Here's how the part is built. I have some questions about the finished solid (model axes, mm). A direction names the side the tool comes from. Round coordinates to 2 decimals unless told otherwise and drop trailing zeros. Order: outer loops, then holes, each group sorted by start corner. A loop starts at its lowest first (then second) coordinate and runs counter-clockwise, first axis right, second up.
```python
from build123d import *

# Parameters (mm, degrees)
ESQUISSE1_W             = 165
ESQUISSE1_H             = 276
BOSS_EXTRU_1_DEPTH      = 6
ESQUISSE2_W             = 38
ESQUISSE2_H             = 6
ESQUISSE2_W_2           = 6
ESQUISSE2_H_2           = 32
ESQUISSE2_H_3           = 68
ESQUISSE2_W_3           = 40
EXTERIEUR_DEPTH         = 10
ESQUISSE3_R             = 11
ESQUISSE3_W             = 20
ESQUISSE3_H             = 6
ENL_V_MAT_EXTRU_2_DEPTH = 322.616230934
ESQUISSE4_R             = 1.5
ESQUISSE4_R_2           = 1.252769876
ESQUISSE4_R_3           = 1.193016672
ESQUISSE4_R_4           = 1.226747293
ESQUISSE4_R_5           = 1.185631844
ENL_V_MAT_EXTRU_3_DEPTH = 322.616230934
ESQUISSE5_R             = 2.995
ESQUISSE5_R_2           = 3
ESQUISSE5_R_3           = 2
ENL_V_MAT_EXTRU_4_DEPTH = 3
ESQUISSE6_W             = 20
ESQUISSE6_H             = 100
ENL_V_MAT_EXTRU_5_DEPTH = 322.616230934


with BuildPart() as part:
    # Esquisse1 → Boss.-Extru.1 (new body)
    with BuildSketch(Plane.XY):
        with Locations((-82.5, 138)):
            Rectangle(ESQUISSE1_W, ESQUISSE1_H)
    extrude(amount=BOSS_EXTRU_1_DEPTH)

    # Esquisse2 → exterieur (cut)
    with BuildSketch(Plane.XY.offset(6)):
        with Locations((-86, 273)):
            Rectangle(ESQUISSE2_W, ESQUISSE2_H)
        with Locations((-162, 220)):
            Rectangle(ESQUISSE2_W_2, ESQUISSE2_H_2)
        with Locations((-162, 102)):
            Rectangle(ESQUISSE2_W_2, ESQUISSE2_H_3)
        Polygon((-137, 36), (-137, 6), (-100, 6), (-100, 0), (-165, 0), (-165, 36), align=None)
        with Locations((-40, 3)):
            Rectangle(ESQUISSE2_W_3, ESQUISSE2_H)
    extrude(amount=-EXTERIEUR_DEPTH, mode=Mode.SUBTRACT)

    # Esquisse3 → Enlèv. mat.-Extru.2 (cut, through all)
    with BuildSketch(Plane.XY.offset(6)):
        with Locations((-144, 178.92)):
            Circle(ESQUISSE3_R)
        with Locations((-135, 99)):
            Rectangle(ESQUISSE3_W, ESQUISSE3_H)
    extrude(amount=-ENL_V_MAT_EXTRU_2_DEPTH, mode=Mode.SUBTRACT)

    # Esquisse4 → Enlèv. mat.-Extru.3 (cut, through all)
    with BuildSketch(Plane.XY.offset(6)):
        with Locations((-60, 273)):
            Circle(ESQUISSE4_R)
        with Locations((-112, 273)):
            Circle(ESQUISSE4_R)
        with Locations((-162, 197)):
            Circle(ESQUISSE4_R)
        with Locations((-162, 170)):
            Circle(ESQUISSE4_R)
        with Locations((-162, 143)):
            Circle(ESQUISSE4_R)
        with Locations((-162, 61)):
            Circle(ESQUISSE4_R)
        with Locations((-162, 43)):
            Circle(ESQUISSE4_R)
        with Locations((-93, 3)):
            Circle(ESQUISSE4_R)
        with Locations((-67, 3)):
            Circle(ESQUISSE4_R)
        with Locations((-10, 3)):
            Circle(ESQUISSE4_R)
        with Locations((-162, 269)):
            Circle(ESQUISSE4_R)
        with Locations((-162, 243)):
            Circle(ESQUISSE4_R)
        with Locations((-117.5, 27)):
            Circle(ESQUISSE4_R_2)
        with Locations((-117.5, 43)):
            Circle(ESQUISSE4_R_3)
        with Locations((-101.5, 43)):
            Circle(ESQUISSE4_R_4)
        with Locations((-101.5, 27)):
            Circle(ESQUISSE4_R_5)
        with Locations((-152, 99)):
            Circle(ESQUISSE4_R)
    extrude(amount=-ENL_V_MAT_EXTRU_3_DEPTH, mode=Mode.SUBTRACT)

    # Esquisse5 → Enlèv. mat.-Extru.4 (cut)
    with BuildSketch(Plane(origin=(0, 0, 0), x_dir=(-1, 0, 0), z_dir=(0, 0, -1))):
        with Locations((60, 273)):
            Circle(ESQUISSE5_R)
        with Locations((112, 273)):
            Circle(ESQUISSE5_R)
        with Locations((162, 197)):
            Circle(ESQUISSE5_R)
        with Locations((162, 170)):
            Circle(ESQUISSE5_R)
        with Locations((162, 143)):
            Circle(ESQUISSE5_R)
        with Locations((162, 61)):
            Circle(ESQUISSE5_R)
        with Locations((162, 43)):
            Circle(ESQUISSE5_R)
        with Locations((93, 3)):
            Circle(ESQUISSE5_R)
        with Locations((67, 3)):
            Circle(ESQUISSE5_R)
        with Locations((10, 3)):
            Circle(ESQUISSE5_R)
        with Locations((162, 269)):
            Circle(ESQUISSE5_R)
        with Locations((162, 243)):
            Circle(ESQUISSE5_R)
        with Locations((152, 99)):
            Circle(ESQUISSE5_R_2)
        with Locations((117.5, 43)):
            Circle(ESQUISSE5_R_3)
        with Locations((117.5, 27)):
            Circle(ESQUISSE5_R_3)
        with Locations((101.5, 27)):
            Circle(ESQUISSE5_R_3)
        with Locations((101.5, 43)):
            Circle(ESQUISSE5_R_3)
    extrude(amount=-ENL_V_MAT_EXTRU_4_DEPTH, mode=Mode.SUBTRACT)

    # Esquisse6 → Enlèv. mat.-Extru.5 (cut, through all)
    with BuildSketch(Plane(origin=(0, 0, 0), x_dir=(-1, 0, 0), z_dir=(0, 0, -1))):
        with Locations((107, 121)):
            Rectangle(ESQUISSE6_W, ESQUISSE6_H)
    extrude(amount=-ENL_V_MAT_EXTRU_5_DEPTH, mode=Mode.SUBTRACT)


solid = part.part
```
1) For faces 1 (the flat face through (-163.3, 241.7, 3)), 2 (the flat face through (-135, 276, 3)), 3 (the flat face through (-86, 270, 3)), 4 (the flat face through (-151, 36, 3)), which set-ups out of +Z, -Z, +X, -X, +Y, -Y let a thin tool reach every point of the face, with its end or its side?
2) If we section it at B-B (z = 4.3): Give the number of separate pieces and of enclosed holes in the cut face, plus the area to 3 significant figures.
3) If we section it at A-A (y = 131): Write out the boundary of the cut face in (x, z), plus the area to 3 significant figures.
4) I'm going to push flat-ended pins straight in: pin 1 (3 mm diameter, centred on y = 94, z = 4, fed in from -X); pin 2 (3 mm diameter, centred on x = -161.5, y = 143.5, fed in from -Z); pin 3 (1 mm diameter, centred on x = -38.5, z = 4, fed in from -Y). Where does each tip first touch, or does it pass through?
5) We'd pull the mould along Y, two halves only. Please class faces 5 (the flat face through (-165, 256, 3)), 6 (the flat face through (-61.3, 271.7, 3)), 7 (the flat face through (-40, 6, 3)): +Y half, -Y half, draft (parallel to the pull), parting line (faces both ways), or undercut.
6) I need wall thicknesses on line 1 (X direction, y = 123.5, z = 4.3); line 2 (Y direction, x = -10, z = 4.7); line 3 (X direction, y = 215.5, z = 3.9). Which ranges of each line are inside material? Lowest first, please.
7) If we section it at C-C (x = -75): Write out the boundary of the cut face in (y, z), plus the area to 3 significant figures.
Solutions:
1. face 1: -Z
1. face 2: +Z, -Z, +X, -X, +Y
1. face 3: +Z, -Z, +Y
1. face 4: +Z, -Z, -X, -Y
2. separate pieces: 1
2. enclosed holes: 20
2. area: 40,600 mm2
3. outline: (-159, 0) - (-117, 0) - (-117, 6) - (-159, 6) - close; (-97, 0) - (0, 0) - (0, 6) - (-97, 6) - close
3. area: 834 mm2
4. pin 1: stops at x = -159
4. pin 2: stops at z = 3
4. pin 3: stops at y = 6
5. face 5: draft
5. face 6: undercut
5. face 7: -Y half
6. line 1: x = -159 to -117, -97 to 0
6. line 2: y = 0 to 1.5, 4.5 to 276
6. line 3: x = -159 to 0
7. outline: (0, 0) - (270, 0) - (270, 6) - (0, 6) - close
7. area: 1,620 mm2
